from build123d import *

# Parameters (mm, degrees)
F0_W      = 100
F0_H      = 110
F1_DEPTH  = 3
F3_DEPTH  = 25
F4_W      = 15
F4_H      = 6
F5_DEPTH  = 30
F6_R      = 3
F7_R      = 2.99999
F8_R      = 1.5
F9_DEPTH  = 25
F10_R     = 1.5
F11_DEPTH = 25
F12_R     = 1.5
F13_DEPTH = 25
F14_R     = 1.5
F15_DEPTH = 25


# Not quite as in the source:
# - a fillet or chamfer is up to 0.001 mm smaller than in the source, because OpenCascade refuses the exact size


with BuildPart() as f1:
    # F0 (on Front) → F1 (new body)
    with BuildSketch(Plane.XZ):
        with Locations((50, 55)):
            Rectangle(F0_W, F0_H)
    extrude(amount=F1_DEPTH)

    # F2 (on face) → F3 (cut)
    with BuildSketch(Plane.XZ.offset(3)):
        with BuildLine():
            Line((0, 110), (0, 65))
            ThreePointArc((0, 65), (16.3054104548, 84.5617848231), (17.5, 110))
            Line((17.5, 110), (0, 110))
        make_face()
        with BuildLine():
            Line((100, 110), (82.5, 110))
            ThreePointArc((82.5, 110), (83.6945895452, 84.5617848231), (100, 65))
            Line((100, 65), (100, 110))
        make_face()
        with BuildLine():
            ThreePointArc((100, 45), (83.6945895452, 25.4382151769), (82.5, 0))
            Line((82.5, 0), (100, 0))
            Line((100, 0), (100, 45))
        make_face()
        with BuildLine():
            Line((0, 45), (0, 0))
            Line((0, 0), (17.5, 0))
            ThreePointArc((17.5, 0), (16.3054104548, 25.4382151769), (0, 45))
        make_face()
    extrude(amount=-F3_DEPTH, mode=Mode.SUBTRACT)

    # F4 (on face) → F5 (join)
    with BuildSketch(Plane(origin=(0, 0, 0), x_dir=(-1, 0, 0), z_dir=(0, 1, 0))):
        with Locations((-50, 7)):
            Rectangle(F4_W, F4_H)
    extrude(amount=F5_DEPTH)

    # F6
    f6_edges = [f1.edges().sort_by_distance(p)[0] for p in [
        (50, 30, 4),
    ]]
    fillet(f6_edges, radius=F6_R)

    # F7 (radius 3 in the source; OpenCascade refuses exactly that, so slightly less here)
    f7_edges = [f1.edges().sort_by_distance(p)[0] for p in [
        (50, 30, 10),
    ]]
    fillet(f7_edges, radius=F7_R)

    # F8 (on face) → F9 (cut)
    with BuildSketch(Plane(origin=(0, 0, 0), x_dir=(-1, 0, 0), z_dir=(0, 1, 0))):
        with Locations((-40.1520836353, 6.8762069568)):
            Circle(F8_R)
        with Locations((-60.1520836353, 6.8762069568)):
            Circle(F8_R)
    extrude(amount=-F9_DEPTH, mode=Mode.SUBTRACT)

    # F10 (on face) → F11 (cut)
    with BuildSketch(Plane.XZ.offset(3)):
        with Locations((23.3403220773, 107.6833680272)):
            Circle(F10_R)
        with Locations((76.8845230341, 107.3717549443)):
            Circle(F10_R)
    extrude(amount=-F11_DEPTH, mode=Mode.SUBTRACT)

    # F12 (on face) → F13 (cut)
    with BuildSketch(Plane.XZ.offset(3)):
        with Locations((96.7704804272, 62.8292252972)):
            Circle(F12_R)
        with Locations((97.3125401127, 46.8384100805)):
            Circle(F12_R)
        with Locations((2.5671770603, 62.836966732)):
            Circle(F12_R)
    extrude(amount=-F13_DEPTH, mode=Mode.SUBTRACT)

    # F14 (on face) → F15 (cut)
    with BuildSketch(Plane.XZ.offset(3)):
        with Locations((2.6400329079, 47.0330864191)):
            Circle(F14_R)
    extrude(amount=-F15_DEPTH, mode=Mode.SUBTRACT)


solid = f1.part
Input: part model. Units: mm. Frame: model coordinates. A direction names the side the tool comes from. Coordinates: 2 decimals unless noted, no trailing zeros. Loops run counter-clockwise (first coordinate to the right, second up) from the corner with the lowest first, then second, coordinate; pieces in that order, holes last.
(1) Set-up query: faces 4 (the face through (57.5, 15, 7)), 5 (the face through (50, 13, 4)), 6 (the face through (42.5, 15, 7)). Return all of +Z, -Z, +X, -X, +Y, -Y with unobstructed straight access to the full face (end or side cutting, diameter ignored); none if empty.
(2) Material intervals for probe 1 along Z at (x, y) = (47.5, 13.5); probe 2 along Y at (x, z) = (51, 49.5); probe 3 along X at (y, z) = (3, 8), sorted ascending.
(3) Section B-B on z = 51. Return the cut outline in (x, y), then the cut area to 3 significant figures.
(4) First-contact query: pin 1 Ø1 at (x, z) = (32, 89.5) entering from +Y; pin 2 Ø3 at (y, z) = (9, 5.5) entering from -X; pin 3 Ø8 at (y, z) = (0.5, 56) entering from -X; pin 4 Ø4.5 at (x, y) = (49, 12.5) entering from +Z. Flat tips, straight axial feed; report the tip coordinate or a pass-through.
(5) Pull-direction query (X, two-part tool) for faces 1 (the face through (50, -1, 0)), 2 (the face through (2.31, -1.52, 45.57)), 3 (the face through (83.83, -1.52, 25.78)); classes: released by +X, released by -X, zero draft, split by the parting line, or undercut.
(6) Section A-A on x = 40. Return the cut outline in (y, z).
(7) Section C-C on y = 10.5. Return the cut outline in (x, z), then the cut area to 3 significant figures.
Data:
1. face 4: +Z, -Z, +X, +Y
1. face 5: -Z, +X, -X, +Y
1. face 6: +Z, -Z, -X, +Y
2. probe 1: z = 4 to 10
2. probe 2: y = -3 to 0
2. probe 3: x = 42.5 to 57.5
3. outline: (0, -3) - (100, -3) - (100, 0) - (0, 0) - close
3. area: 300 mm2
4. pin 1: stops at y = 0
4. pin 2: stops at x = 42.5
4. pin 3: stops at x = 0
4. pin 4: stops at z = 10
5. face 1: zero draft
5. face 2: undercut
5. face 3: released by +X
6. outline: (-3, 0) - (0, 0) - (0, 5.38) - (-3, 5.38) - close; (-3, 8.37) - (0, 8.37) - (0, 110) - (-3, 110) - close
7. outline: (42.5, 4) - (57.5, 4) - (57.5, 10) - (42.5, 10) - close
7. area: 90.0 mm2
